from build123d import *

# Parameters (mm, degrees)
SKETCH1_W            = 111
SKETCH1_H            = 126
BOSS_EXTRUDE1_DEPTH  = 6
SKETCH2_W            = 216
SKETCH2_H            = 111
BOSS_EXTRUDE2_DEPTH  = 6
SKETCH3_W            = 216
SKETCH3_H            = 132
BOSS_EXTRUDE3_DEPTH  = 6
SKETCH5_W            = 216
SKETCH5_H            = 99.986345045
CUT_EXTRUDE1_DEPTH   = 75
SKETCH7_W            = 216
SKETCH7_H            = 99.986345045
BOSS_EXTRUDE4_DEPTH  = 5
CUT_EXTRUDE2_DEPTH   = 314
SKETCH9_W            = 85.5
SKETCH9_H            = 55
CUT_EXTRUDE3_DEPTH   = 14
FILLET1_R            = 15
CUT_EXTRUDE4_DEPTH   = 27
SKETCH11_W           = 65
SKETCH11_H           = 16.2
CUT_EXTRUDE5_DEPTH   = 2
SKETCH12_W           = 3.5
SKETCH12_H           = 12
CUT_EXTRUDE6_DEPTH   = 11
BOSS_EXTRUDE5_DEPTH  = 6
SKETCH22_R           = 1.5
CUT_EXTRUDE13_DEPTH  = 20
BOSS_EXTRUDE6_DEPTH  = 15
SKETCH25_R           = 1.5
CUT_EXTRUDE14_DEPTH  = 15
BOSS_EXTRUDE9_START  = -6
BOSS_EXTRUDE9_DEPTH  = 6
SKETCH35_W           = 210
SKETCH35_H           = 6
SKETCH35_R           = 1.5
BOSS_EXTRUDE10_DEPTH = 15
SKETCH36_R           = 4
CUT_EXTRUDE16_DEPTH  = 15
SKETCH37_R           = 4
CUT_EXTRUDE17_DEPTH  = 15


with BuildPart() as part:
    # Sketch1 → Boss-Extrude1 (new body)
    with BuildSketch(Plane(origin=(0, 0, 0), x_dir=(0, 0, -1), z_dir=(1, 0, 0))):
        with Locations((55.5, 63)):
            Rectangle(SKETCH1_W, SKETCH1_H)
    extrude(amount=BOSS_EXTRUDE1_DEPTH)

    # Sketch2 → Boss-Extrude2 (add)
    with BuildSketch(Plane(origin=(0, 126, 0), x_dir=(1, 0, 0), z_dir=(0, 1, 0))):
        with Locations((108, 55.5)):
            Rectangle(SKETCH2_W, SKETCH2_H)
    extrude(amount=BOSS_EXTRUDE2_DEPTH)

    # Sketch3 → Boss-Extrude3 (add)
    with BuildSketch(Plane.XY):
        with Locations((108, 66)):
            Rectangle(SKETCH3_W, SKETCH3_H)
    extrude(amount=BOSS_EXTRUDE3_DEPTH)

    # Sketch5 → Cut-Extrude1 (cut)
    with BuildSketch(Plane(origin=(0, 19.268574279, 27.51837595), x_dir=(1, 0, 0), z_dir=(0, -0.5735764363510416, -0.8191520442889949))):
        with Locations((108, -87.509316119)):
            Rectangle(SKETCH5_W, SKETCH5_H)
    extrude(amount=-CUT_EXTRUDE1_DEPTH, mode=Mode.SUBTRACT)

    # Sketch7 → Boss-Extrude4 (add)
    with BuildSketch(Plane(origin=(0, 19.268574279, 27.51837595), x_dir=(1, 0, 0), z_dir=(0, -0.5735764363510416, -0.8191520442889949))):
        with Locations((108, -87.509316119)):
            Rectangle(SKETCH7_W, SKETCH7_H)
    extrude(amount=-BOSS_EXTRUDE4_DEPTH)

    # Sketch8 → Cut-Extrude2 (cut)
    with BuildSketch(Plane(origin=(216, 0, 0), x_dir=(0, 0, -1), z_dir=(1, 0, 0))):
        Polygon((-6, 50), (-6, 58.717233978), (-10.095760221, 52.867882182), align=None)
        Polygon((51.212736322, 132), (45.313145189, 132), (47.254051253, 134.771901126), align=None)
    extrude(amount=-CUT_EXTRUDE2_DEPTH, mode=Mode.SUBTRACT)

    # Sketch9 → Cut-Extrude3 (cut)
    with BuildSketch(Plane(origin=(0, 22.136456461, 31.614136171), x_dir=(1, 0, 0), z_dir=(0, 0.5735764363510417, 0.8191520442889949))):
        with Locations((108, 89.387752907)):
            Rectangle(SKETCH9_W, SKETCH9_H)
    extrude(amount=-CUT_EXTRUDE3_DEPTH, mode=Mode.SUBTRACT)

    # Fillet1
    fillet1_edges = [part.edges().sort_by_distance(p)[0] for p in [
        (111, 58.56888804, 0),
        (108, 58.717233978, 6),
    ]]
    fillet(fillet1_edges, radius=FILLET1_R)

    # Sketch10 → Cut-Extrude4 (cut)
    with BuildSketch(Plane.ZY):
        with BuildLine():
            Line((-87.5, 42.5), (-17.5, 42.5))
            ThreePointArc((-17.5, 42.5), (-10, 35), (-17.5, 27.5))
            Line((-17.5, 27.5), (-87.5, 27.5))
            ThreePointArc((-87.5, 27.5), (-95, 35), (-87.5, 42.5))
        make_face()
        with BuildLine():
            Line((-89.152421831, 99.5), (-39.152421831, 99.5))
            ThreePointArc((-39.152421831, 99.5), (-31.652421831, 92), (-39.152421831, 84.5))
            Line((-39.152421831, 84.5), (-89.152421831, 84.5))
            ThreePointArc((-89.152421831, 84.5), (-96.652421831, 92), (-89.152421831, 99.5))
        make_face()
    extrude(amount=-CUT_EXTRUDE4_DEPTH, mode=Mode.SUBTRACT)

    # Sketch11 → Cut-Extrude5 (cut)
    with BuildSketch(Plane.XY.offset(6)):
        with Locations((108, 26.993876072)):
            Rectangle(SKETCH11_W, SKETCH11_H)
    extrude(amount=-CUT_EXTRUDE5_DEPTH, mode=Mode.SUBTRACT)

    # Sketch12 → Cut-Extrude6 (cut)
    with BuildSketch(Plane.XY.offset(4)):
        with Locations((86.25, 26.993876072)):
            Rectangle(SKETCH12_W, SKETCH12_H)
        with Locations((94.75, 26.993876072)):
            Rectangle(SKETCH12_W, SKETCH12_H)
        with Locations((103.75, 26.993876072)):
            Rectangle(SKETCH12_W, SKETCH12_H)
        with Locations((112.25, 26.993876072)):
            Rectangle(SKETCH12_W, SKETCH12_H)
        with Locations((121.25, 26.993876072)):
            Rectangle(SKETCH12_W, SKETCH12_H)
        with Locations((129.75, 26.993876072)):
            Rectangle(SKETCH12_W, SKETCH12_H)
    extrude(amount=-CUT_EXTRUDE6_DEPTH, mode=Mode.SUBTRACT)

    # Sketch13 → Boss-Extrude5 (add)
    with BuildSketch(Plane(origin=(216, 0, 0), x_dir=(0, 0, -1), z_dir=(1, 0, 0))):
        with BuildLine():
            Line((111, 126), (111, 132))
            Line((111, 132), (45.313145189, 132))
            Line((45.313145189, 132), (-3.287280664, 62.59139869))
            ThreePointArc((-3.287280664, 62.59139869), (-5.305754261, 58.498339137), (-6, 53.987752145))
            Line((-6, 53.987752145), (-6, 0))
            Line((-6, 0), (0, 0))
            Line((0, 0), (0, 53.839406207))
            ThreePointArc((0, 53.839406207), (0.694245739, 58.3499932), (2.712719336, 62.443052753))
            Line((2.712719336, 62.443052753), (47.215772904, 126))
            Line((47.215772904, 126), (111, 126))
        make_face()
    extrude(amount=BOSS_EXTRUDE5_DEPTH)

    # Sketch22 → Cut-Extrude13 (cut)
    with BuildSketch(Plane.XY.offset(6)):
        with Locations((207, 3)):
            Circle(SKETCH22_R)
        with Locations((192, 3)):
            Circle(SKETCH22_R)
    extrude(amount=-CUT_EXTRUDE13_DEPTH, mode=Mode.SUBTRACT)

    # Sketch24 → Boss-Extrude6 (add)
    with BuildSketch(Plane(origin=(0, 0, -111), x_dir=(-1, 0, 0), z_dir=(0, 0, -1))):
        Polygon((-222, 132), (-222, 126), (-6, 126), (-6, 0), (0, 0), (0, 132), align=None)
    extrude(amount=BOSS_EXTRUDE6_DEPTH)

    # Sketch25 → Cut-Extrude14 (cut)
    with BuildSketch(Plane(origin=(0, 132, 0), x_dir=(1, 0, 0), z_dir=(0, 1, 0))):
        with Locations(Location((21, 123, 0), (0, 0, 270))):
            Circle(SKETCH25_R)
        with Locations(Location((36, 123, 0), (0, 0, 270))):
            Circle(SKETCH25_R)
    extrude(amount=-CUT_EXTRUDE14_DEPTH, mode=Mode.SUBTRACT)

    # Sketch34 → Boss-Extrude9 (add)
    with BuildSketch(Plane(origin=(222, 0, 0), x_dir=(0, 0, -1), z_dir=(1, 0, 0)).offset(BOSS_EXTRUDE9_START)):
        with BuildLine():
            Line((2.712719336, 62.443052753), (47.215772904, 126))
            Line((47.215772904, 126), (62.215772904, 126))
            Line((62.215772904, 126), (17.712719336, 62.443052753))
            ThreePointArc((17.712719336, 62.443052753), (15.694245739, 58.3499932), (15, 53.839406207))
            Line((15, 53.839406207), (15, 0))
            Line((15, 0), (0, 0))
            Line((0, 0), (0, 53.839406207))
            ThreePointArc((0, 53.839406207), (0.694245739, 58.3499932), (2.712719336, 62.443052753))
        make_face()
    extrude(amount=BOSS_EXTRUDE9_DEPTH)

    # Sketch35 → Boss-Extrude10 (add)
    with BuildSketch(Plane(origin=(0, 0, 0), x_dir=(-1, 0, 0), z_dir=(0, 0, -1))):
        with Locations((-111, 3)):
            Rectangle(SKETCH35_W, SKETCH35_H)
        with Locations(Location((-207, 3, 0), (0, 0, 180))):
            Circle(SKETCH35_R, mode=Mode.SUBTRACT)
        with Locations(Location((-192, 3, 0), (0, 0, 180))):
            Circle(SKETCH35_R, mode=Mode.SUBTRACT)
    extrude(amount=BOSS_EXTRUDE10_DEPTH)

    # Sketch36 → Cut-Extrude16 (cut)
    with BuildSketch(Plane(origin=(0, 22.136456461, 31.614136171), x_dir=(1, 0, 0), z_dir=(0, 0.5735764363510417, 0.8191520442889949))):
        with Locations(Location((187.47755458, 89.387752907, 0), (0, 0, 270))):
            Circle(SKETCH36_R)
    extrude(amount=-CUT_EXTRUDE16_DEPTH, mode=Mode.SUBTRACT)

    # Sketch37 → Cut-Extrude17 (cut)
    with BuildSketch(Plane(origin=(0, 22.136456461, 31.614136171), x_dir=(1, 0, 0), z_dir=(0, 0.5735764363510417, 0.8191520442889949))):
        with Locations(Location((32.625, 89.387752907, 0), (0, 0, 270))):
            Circle(SKETCH37_R)
    extrude(amount=-CUT_EXTRUDE17_DEPTH, mode=Mode.SUBTRACT)


solid = part.part
Read the model definition and answer for the solid it produces. Units are mm, in the model's axes. A direction names the side the tool comes from. Round coordinates to 2 decimals unless told otherwise and drop trailing zeros. Order: outer loops, then holes, each group sorted by start corner. A loop starts at its lowest first (then second) coordinate and runs counter-clockwise, first axis right, second up.
1) The part is cut by section A-A on z = -77. Write down the section's boundary in (x, y), plus the area to 3 significant figures.
2) The mould has two halves that part along Y. Classify faces 5 (the face through (3, 84.5, -64)), 6 (the face through (109, 39, 6)), 7 (the face through (218.958, 58.411, -15.714)): released by +Y, released by -Y, zero draft, split by the parting line, or undercut.
3) Straight lines are drawn through the part: L1, parallel to X at y = 129.8, z = -123; L2, parallel to X at y = 3, z = 0; L3, parallel to Y at x = 123, z = -10.5. For each, find the intervals that lie inside material, in ascending order.
4) Flat-ended cylindrical pins translate along their axes: pin 1 (5 mm diameter, centred on x = 149, y = 66.5, fed in from -Z); pin 2 (1 mm diameter, centred on x = 110, z = -42, fed in from -Y); pin 3 (1.5 mm diameter, centred on x = 157, y = 39.5, fed in from -Z). Find the tip coordinate at first contact, or state that the pin passes through.
5) The part is cut by section B-B on y = 75.5. Write down the section's boundary in (x, z), plus the area to 3 significant figures.
6) For faces 1 (the face through (139, 5, -15)), 2 (the face through (216, 66, -20)), 3 (the face through (3, 27.5, -52)), 4 (the face through (116, 126, -86)), determine the directions among +Z, -Z, +X, -X, +Y, -Y from which every point of the face is accessible in a straight line to the end or side of a thin tool.
Resolved:
1. outline: (0, 0) - (6, 0) - (6, 27.5) - (0, 27.5) - close; (0, 42.5) - (6, 42.5) - (6, 84.5) - (0, 84.5) - close; (0, 99.5) - (6, 99.5) - (6, 126) - (222, 126) - (222, 132) - (0, 132) - close
1. area: 1,910 mm2
2. face 5: undercut
2. face 6: zero draft
2. face 7: released by -Y
3. L1: x = 0 to 19.5, 22.5 to 34.5, 37.5 to 222
3. L2: x = 0 to 190.5, 193.5 to 205.5, 208.5 to 222
3. L3: y = 0 to 6
4. pin 1: stops at z = -7.3
4. pin 2: stops at y = 117.84
4. pin 3: stops at z = 0
5. outline: (0, -126) - (6, -126) - (6, -11.86) - (65.25, -11.86) - (65.25, -5.75) - (0, -5.75) - close; (150.75, -11.86) - (216, -11.86) - (216, -26.86) - (222, -26.86) - (222, -5.75) - (150.75, -5.75) - close
5. area: 1,610 mm2
6. face 1: -Z, +X, -Y
6. face 2: -Z
6. face 3: +X, -X
6. face 4: -Z, -Y
